from build123d import *

# Parameters (mm, degrees)
F1_DEPTH = 7.874
F2_DEPTH = 14.224
F3_DEPTH = 12.7
F0_W     = 6.35
F0_H     = 28.448
F4_DEPTH = 7.874
F5_DEPTH = 3.048


with BuildPart() as f1:
    # F0 (on Front) → F1 (new body, symmetric)
    with BuildSketch(Plane.XZ):
        Polygon((6.35, 44.45), (6.35, 16.002), (69.596, 16.002), (83.2485, 26.924), (69.596, 26.924), (69.596, 44.45), align=None)
        with BuildLine():
            ThreePointArc((24.638, 30.226), (26.274687, 34.177313), (30.226, 35.814))
            Line((30.226, 35.814), (54.102, 35.814))
            ThreePointArc((54.102, 35.814), (58.053313, 34.177313), (59.69, 30.226))
            ThreePointArc((59.69, 30.226), (58.053313, 26.274687), (54.102, 24.638))
            Line((54.102, 24.638), (30.226, 24.638))
            ThreePointArc((30.226, 24.638), (26.274687, 26.274687), (24.638, 30.226))
        make_face(mode=Mode.SUBTRACT)
    extrude(amount=F1_DEPTH, both=True)

    # F0 (on Front) → F2 (join, symmetric)
    with BuildSketch(Plane.XZ):
        Polygon((0, 16.002), (0, 0), (0, -16.002), (6.35, -16.002), (69.596, -16.002), (69.596, 0), (69.596, 16.002), (6.35, 16.002), align=None)
    extrude(amount=F2_DEPTH, both=True)

    # F0 (on Front) → F3 (join, symmetric)
    with BuildSketch(Plane.XZ):
        Polygon((69.596, 26.924), (83.2485, 26.924), (105.156, 44.45), (69.596, 44.45), align=None)
    extrude(amount=F3_DEPTH, both=True)

    # F0 (on Front) → F4 (join)
    with BuildSketch(Plane.XZ):
        with Locations((3.175, 30.226)):
            Rectangle(F0_W, F0_H)
    extrude(amount=-F4_DEPTH)

    # F0 (on Front) → F5 (join)
    with BuildSketch(Plane.XZ):
        with Locations((3.175, 30.226)):
            Rectangle(F0_W, F0_H)
    extrude(amount=F5_DEPTH)

    # F6: F1 across plane


with BuildPart() as f1_1:
    add(f1.part)
    add(f1.part.mirror(Plane.XY))


solid = f1_1.part
Design review of the part built by this model. Coordinates are the model's own, in mm. A direction names the side the tool comes from. Coordinates: 2 decimals unless noted, no trailing zeros. Write each loop counter-clockwise with the first axis right and the second up, starting at its lowest first coordinate (ties: lowest second). Pieces come first, ordered by that corner, then holes. Notation, with made-up numbers: (9.5, 80.5) -> (38.5, 80.5) arc R15 ccw to (38.5, 105.5) -> close; hole circle Ø2 at (69, 82). An arc over 180 degrees is marked (long way). Write each question's results on one line, items separated by ' | '. Start each with the question number.
(1) Take a section at C-C on y = 11.5. Write out the cut boundary in (x, z), and give its area (3 significant figures).
(2) The part is to be moulded in two halves that separate along Z. For faces 6 (the face through (69.596, 10, -36)), 7 (the face through (64, 0, -44.45)), 8 (the face through (91.08, -0.18, -33.19)), 9 (the face through (42, 0, -24.638)), say which applies: pulls with the +Z half, pulls with the -Z half, needs draft (parallel to the pull), parting line crosses it, or undercut.
(3) Take a section at A-A on y = -5.5. Write out the cut boundary in (x, z).
(4) Take a section at B-B on x = 35. Write out the cut boundary in (y, z).
(5) Tool access review of faces 1 (the face through (69.596, 10, 36)), 2 (the face through (76, -10, 26.924)), 3 (the face through (76, 10, 26.924)), 4 (the face through (42, 0, 24.638)), 5 (the face through (3, -3.048, 30)): name each direction out of +Z, -Z, +X, -X, +Y, -Y from which nothing blocks a thin tool from reaching the whole face with its end or side.
(6) For line 1 along Z through (x, y) = (92.5, -12.25); line 2 along X through (y, z) = (-11.25, 3); line 3 along Z through (x, y) = (29.5, 12.5), list the stretches that pass through material, from the lowest coordinate up. Write a range as from..to.
(7) Take a section at D-D on z = 32. Write out the cut boundary in (x, y).
(8) Clearance check with flat-ended pins moving along their axes: P1, Ø7, axis at x = 3, z = 28, coming from the -Y side; P2, Ø6, axis at x = 66.5, z = 20, coming from the +Y side; P3, Ø5, axis at x = 2.5, z = -29, coming from the -Y side; P4, Ø2, axis at y = -11, z = -1, coming from the -X side. State where each tip first meets the part, or that it passes through.
Results found:
1) outline: (0, -16) -> (69.6, -16) -> (69.6, 16) -> (0, 16) -> close; (69.6, -44.45) -> (105.16, -44.45) -> (83.25, -26.92) -> (69.6, -26.92) -> close; (69.6, 26.92) -> (83.25, 26.92) -> (105.16, 44.45) -> (69.6, 44.45) -> close | area: 3,090 mm2
2) face 6: needs draft | face 7: pulls with the -Z half | face 8: undercut | face 9: undercut
3) outline: (0, -16) -> (6.35, -16) -> (6.35, -44.45) -> (105.16, -44.45) -> (69.6, -16) -> (69.6, 16) -> (105.16, 44.45) -> (6.35, 44.45) -> (6.35, 16) -> (0, 16) -> close; hole (24.64, -30.23) arc R5.59 ccw to (30.23, -35.81) -> (54.1, -35.81) arc R5.59 ccw to (59.69, -30.23) arc R5.59 ccw to (54.1, -24.64) -> (30.23, -24.64) arc R5.59 ccw to start; hole (24.64, 30.23) arc R5.59 ccw to (30.23, 24.64) -> (54.1, 24.64) arc R5.59 ccw to (59.69, 30.23) arc R5.59 ccw to (54.1, 35.81) -> (30.23, 35.81) arc R5.59 ccw to start
4) outline: (-14.22, -16) -> (-7.87, -16) -> (-7.87, -24.64) -> (7.87, -24.64) -> (7.87, -16) -> (14.22, -16) -> (14.22, 16) -> (7.87, 16) -> (7.87, 24.64) -> (-7.87, 24.64) -> (-7.87, 16) -> (-14.22, 16) -> close; (-7.87, -44.45) -> (7.87, -44.45) -> (7.87, -35.81) -> (-7.87, -35.81) -> close; (-7.87, 35.81) -> (7.87, 35.81) -> (7.87, 44.45) -> (-7.87, 44.45) -> close
5) face 1: +Z, -X, +Y | face 2: +X, -X, -Y | face 3: +X, -X, +Y | face 4: +Y, -Y | face 5: +Z, -X, -Y
6) line 1: z = -44.45..-34.33, 34.33..44.45 | line 2: x = 0..69.6 | line 3: z = -16..16
7) outline: (0, -3.05) -> (6.35, -3.05) -> (6.35, -7.87) -> (24.93, -7.87) -> (24.93, 7.87) -> (0, 7.87) -> close; (59.4, -7.87) -> (69.6, -7.87) -> (69.6, -12.7) -> (89.59, -12.7) -> (89.59, 12.7) -> (69.6, 12.7) -> (69.6, 7.87) -> (59.4, 7.87) -> close
8) P1: stops at y = -7.87 | P2: stops at y = 7.87 | P3: stops at y = -3.05 | P4: stops at x = 0
